Part print with two shaded views. Sizes in mm from the minimum x, y, z corner. A direction names the side the tool comes from. Give positions to 0.01 mm unless a question says otherwise; leave off trailing zeros. Write each loop counter-clockwise with the first axis right and the second up, starting at its lowest first coordinate (ties: lowest second). Pieces come first, ordered by that corner, then holes. Notation, with made-up numbers: (65.25, 45) -> (84.25, 45) arc R21 ccw to (84.25, 72) -> close; hole circle Ø10 at (47.25, 88). An arc over 180 degrees is marked (long way). Answer in a Markdown table with one row per item. Add a question column.
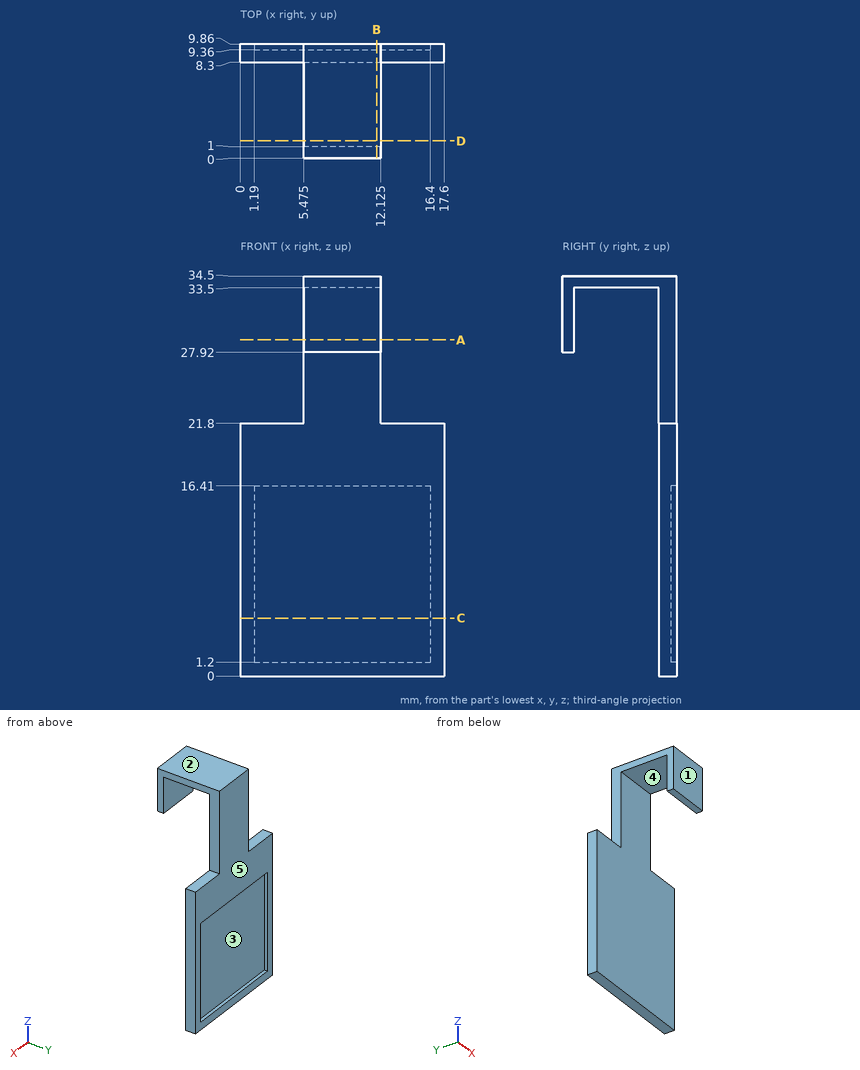
Item 1: Probe L1, parallel to Y at x = 0.5, z = 9; L2, parallel to Y at x = 14.75, z = 8; L3, parallel to Y at x = 9.25, z = 30.5. List the from-to ranges inside material, lowest first. Write a range as from..to.
Item 2: Slice it at D-D, the plane y = 1.5. List the corners of the cut face in (x, z) (3 decimals), then the cut area to 3 significant figures.
Item 3: Mould opens along Z. For the marked faces 1, 2 and 3 say: released by +Z, released by -Z, zero draft, split by the parting line, or undercut.
Item 4: Slice it at B-B, the plane x = 11.75. List the corners of the cut face in (y, z).
Item 5: Which spindle directions (+Z, -Z, +X, -X, +Y, -Y) get a long thin tool onto all of the face, cutting with end or side? Do the marked faces 4 and 5. Say none if no direction does.
Item 6: Drop flat-ended pins along their axis: pin 1 Ø0.8 at (x, y) = (15.5, 9.5) entering from +Z; pin 2 Ø5.5 at (x, y) = (7.5, 3) entering from -Z; pin 3 Ø8 at (x, z) = (10.5, 22.5) entering from -Y. Give the stop position or say it passes through.
Item 7: Slice it at C-C, the plane z = 5. List the corners of the cut face in (x, y).
Item 8: Slice it at A-A, the plane z = 29. List the corners of the cut face in (x, y) (3 decimals).
Answer key:
| question | item | result |
|---|---|---|
| 1 | L1 | y = 8.3..9.86 |
| 1 | L2 | y = 8.3..9.36 |
| 1 | L3 | y = 0..1, 8.3..9.86 |
| 2 | outline | (5.475, 33.5) -> (12.125, 33.5) -> (12.125, 34.5) -> (5.475, 34.5) -> close |
| 2 | area | 6.65 mm² |
| 3 | face 1 | zero draft |
| 3 | face 2 | released by +Z |
| 3 | face 3 | undercut |
| 4 | outline | (0, 27.92) -> (1, 27.92) -> (1, 33.5) -> (8.3, 33.5) -> (8.3, 0) -> (9.86, 0) -> (9.86, 1.2) -> (9.36, 1.2) -> (9.36, 16.41) -> (9.86, 16.41) -> (9.86, 34.5) -> (0, 34.5) -> close |
| 5 | face 4 | -Z, +X, -X |
| 5 | face 5 | +Z, -Z, +X, -X, +Y |
| 6 | pin 1 | stops at z = 21.8 |
| 6 | pin 2 | stops at z = 27.92 |
| 6 | pin 3 | stops at y = 8.3 |
| 7 | outline | (0, 8.3) -> (17.6, 8.3) -> (17.6, 9.86) -> (16.4, 9.86) -> (16.4, 9.36) -> (1.19, 9.36) -> (1.19, 9.86) -> (0, 9.86) -> close |
| 8 | outline | (5.475, 0) -> (12.125, 0) -> (12.125, 1) -> (5.475, 1) -> close; (5.475, 8.3) -> (12.125, 8.3) -> (12.125, 9.86) -> (5.475, 9.86) -> close |
